Source: CAD feature listing. Evaluate the final solid. Frame: model axes, mm. Face numbers are marked on the shaded views. Round coordinates to 2 decimals unless told otherwise and drop trailing zeros. Loops run counter-clockwise (first coordinate to the right, second up) from the corner with the lowest first, then second, coordinate; pieces in that order, holes last. Notation, with made-up numbers: (-1.5, 22.25) -> (20.5, 22.25) arc R21 ccw to (20.5, 58.25) -> close; hole circle Ø1 at (-22.75, 46). An arc over 180 degrees is marked (long way). Write item = value, one per line.
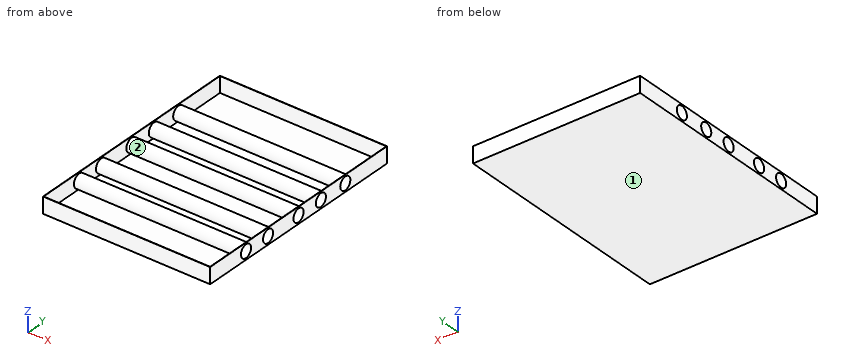
from build123d import *

# Parameters (mm, degrees)
F0_W     = 1320.8
F0_H     = 127
F1_DEPTH = 1778
F2_R     = 50.8
F3_DEPTH = 1465.58
F4_T     = -2.54


with BuildPart() as f1:
    # F0 (on Front) → F1 (new body)
    with BuildSketch(Plane.XZ):
        with Locations((-660.4, 63.5)):
            Rectangle(F0_W, F0_H)
    extrude(amount=-F1_DEPTH)

    # F2 (on face) → F3 (cut)
    with BuildSketch(Plane(origin=(-1320.8, 0, 0), x_dir=(0, -1, 0), z_dir=(-1, 0, 0))):
        with Locations((-1358.689666, 63.5)):
            Circle(F2_R)
        with Locations((-888.521751, 63.5)):
            Circle(F2_R)
        with Locations((-360.66384, 63.5)):
            Circle(F2_R)
        with Locations((-582.459867, 63.5)):
            Circle(F2_R)
        with Locations((-1113.455415, 63.5)):
            Circle(F2_R)
    extrude(amount=-F3_DEPTH, mode=Mode.SUBTRACT)

    # F4
    f4_openings = [f1.faces().sort_by_distance(p)[0] for p in [
        (-660.4, 889, 127),
    ]]
    offset(amount=F4_T, openings=f4_openings)


solid = f1.part
1. Mould query, pull axis Y, two halves, no side actions, for the marked faces 1 and 2. Classes: released by +Y, released by -Y, zero draft, split by the parting line, or undercut.
Evaluation:
face_1 = zero draft
face_2 = undercut
2. Contact query for flat-ended pins moving along their axis: pin 1 Ø6 at (x, z) = (-1001, 22.5) entering from -Y; pin 2 Ø1 at (x, y) = (-672, 420.5) entering from +Z; pin 3 Ø10 at (x, y) = (-977.5, 1405.5) entering from +Z; pin 4 Ø8 at (x, y) = (-836, 309.5) entering from +Z. Output: stop coordinate, or through.
Evaluation:
pin_1 = 0
pin_2 = 2.54
pin_3 = 96.62
pin_4 = 88.41
3. Section query A-A (x = -985). Give the number of separate pieces and of enclosed holes in the cut face, then the cut area to 3 significant figures.
Evaluation:
separate_pieces = 6
enclosed_holes = 5
area = 9,300 mm²
4. Line query: probe 1 along X at (y, z) = (393, 9); probe 2 along Z at (x, y) = (-404, 1135); probe 3 along Z at (x, y) = (-1000, 697.5). Output: solid intervals per line, ascending. Write a range as from..to.
Evaluation:
probe_1 = -1320.8..-1318.26, -2.54..0
probe_2 = 0..2.54, 14.7..17.49, 109.51..112.3
probe_3 = 0..2.54
5. Section query C-C (y = 754). Return the cut outline in (x, z), then the cut area to 3 significant figures.
Evaluation:
outline = (-1320.8, 0) -> (0, 0) -> (0, 127) -> (-2.54, 127) -> (-2.54, 2.54) -> (-1318.26, 2.54) -> (-1318.26, 127) -> (-1320.8, 127) -> close
area = 3,990 mm²
